The listing builds one solid part. Answer for the finished solid, in the listing's coordinates (mm). A direction names the side the tool comes from. Round coordinates to 2 decimals unless told otherwise and drop trailing zeros. Write each loop counter-clockwise with the first axis right and the second up, starting at its lowest first coordinate (ties: lowest second). Pieces come first, ordered by that corner, then holes.
Item 1: Find the intervals of material crossed by probe 1 along Z at (x, y) = (57, 34); probe 2 along Y at (x, z) = (39.5, 16); probe 3 along X at (y, z) = (37.5, -16.5), in increasing order.
Item 2: Each of these flat-tipped pins is pushed along its axis until it touches: pin 1 (11 mm diameter, centred on y = 31, z = -17, fed in from +X); pin 2 (10.5 mm diameter, centred on x = 34, y = 20.5, fed in from -Z). Where does it stop, or does it pass through?
Item 3: A tool of negligible diameter and unlimited length cuts with its end or side. For faces 4 (the face through (41.21, 50.86, 15.49)), 5 (the face through (43, 40.647, -15)), from which of +Z, -Z, +X, -X, +Y, -Y can it reach the whole face along a straight path? Write none if from no direction.
Item 4: Find section A-A on x = 54.5. Give the vertices of the cut face in (y, z), then the cut area to 3 significant figures.
Item 5: For a pull along Y with two mould halves and no side action, classify faces 1 (the face through (44, 0, 15)), 2 (the face through (70.262, 23, -15)), 3 (the face through (44, 95.795, 15)) as +Y half, -Y half, draft (parallel to the pull), parting line (faces both ways), or undercut.
```python
from build123d import *

# Parameters (mm, degrees)
F0_W          = 89.2122089863
F0_H          = 95.7951173186
F1_DEPTH      = 20
F1_DEPTH_BACK = 50
F2_T1_DEPTH   = 145.7951173186
F4_D          = 4.2
F5_W          = 53.7064000964
F5_H          = 35.0269903429
F6_DEPTH      = 10


# Not quite as in the source:
# - a fillet or chamfer that OpenCascade refuses, or shapes differently, is made with other operations: its cross-section is extruded or revolved along the edge and cut away or added


with BuildPart() as f1:
    # F0 (on Top) → F1 (new body, two sides)
    with BuildSketch(Plane.XY) as f1_sk:
        with Locations((44.6061044931, 47.8975586593)):
            Rectangle(F0_W, F0_H)
    extrude(amount=-F1_DEPTH)
    extrude(f1_sk.sketch, amount=F1_DEPTH_BACK)

    # F2: fillet of radius 10 on 1 edges, made by hand

    # F2_s2 → F2_t1 (cut)
    with BuildSketch(Plane.XZ.offset(-120.7951173186)):
        with BuildLine():
            add(Edge.make_bspline(
                [(89.2122089863, -10), (89.2122089863, -20), (79.2122089863, -20)],
                knots=[0, 0, 0, 1, 1, 1], degree=2, weights=[1, 0.1111111111, 1]))
            Line((79.2122089863, -20), (89.2122089863, -20))
            Line((89.2122089863, -20), (89.2122089863, -10))
        make_face()
    extrude(amount=F2_T1_DEPTH, mode=Mode.SUBTRACT)

    # F4 (through all)
    with Locations(Plane(origin=(0, 0, -20), x_dir=(1, 0, 0), z_dir=(0, 0, -1))):
        with Locations((40.9390032291, -52.9426522553)):
            Hole(F4_D / 2)

    # F5 (on face) → F6 (cut)
    with BuildSketch(Plane(origin=(0, 0, -20), x_dir=(1, 0, 0), z_dir=(0, 0, -1))):
        with Locations((43.4090383351, -23.1333931442)):
            Rectangle(F5_W, F5_H)
    extrude(amount=-F6_DEPTH, mode=Mode.SUBTRACT)


solid = f1.part
```
Check values:
1. probe 1: z = -10 to 50
1. probe 2: y = 0 to 51.41, 54.47 to 95.8
1. probe 3: x = 0 to 16.56, 70.26 to 83.69
2. pin 1: stops at x = 88.32
2. pin 2: stops at z = -10
3. face 4: +Z, -Z
3. face 5: -Z
4. outline: (0, -20) - (5.62, -20) - (5.62, -10) - (40.65, -10) - (40.65, -20) - (95.8, -20) - (95.8, 50) - (0, 50) - close
4. area: 6,360 mm2
5. face 1: -Y half
5. face 2: undercut
5. face 3: +Y half
